from build123d import *

# Parameters (mm, degrees)
F0_R     = 10
F1_DEPTH = 1.5
F2_R     = 9
F3_DEPTH = 24
F4_R     = 7
F5_DEPTH = 25.501


with BuildPart() as f1:
    # F0 (on Top) → F1 (new body)
    with BuildSketch(Plane.XY):
        Circle(F0_R)
    extrude(amount=-F1_DEPTH)

    # F2 (on face) → F3 (join)
    with BuildSketch(Plane(origin=(0, 0, -1.5), x_dir=(1, 0, 0), z_dir=(0, 0, -1))):
        Circle(F2_R)
    extrude(amount=F3_DEPTH)

    # F4 (on face) → F5 (cut, through all)
    with BuildSketch(Plane.XY):
        Circle(F4_R)
    extrude(amount=-F5_DEPTH, mode=Mode.SUBTRACT)


solid = f1.part
Geometry: final body of the model. Coordinates: model frame, mm. Coordinates: 2 decimals unless noted, no trailing zeros. Order: outer loops, then holes, each group sorted by start corner. A loop starts at its lowest first (then second) coordinate and runs counter-clockwise, first axis right, second up. Notation, with made-up numbers: M 84.25,60.5 L 99.25,60.5 A18 ccw 99.25,70.5 Z; hole C 47.25,53.5 d2. An arc over 180 degrees is marked long. One line per question, with ' | ' between items. Start each with the question number.
Item 1: Cut plane C-C, the plane z = -8.5. Return the cut outline in (x, y), then the cut area to 3 significant figures.
Item 2: Cut plane B-B, the plane x = -4.25. Return the cut outline in (y, z).
Item 3: Ray query, probe 1 along Y at (x, z) = (0, -9); probe 2 along X at (y, z) = (5.5, -9.5); probe 3 along Z at (x, y) = (-9, 1). Return the intervals inside material, ascending. Write a range as [from, to].
Item 4: Pin query (flat end, axial travel): pin 1 Ø6 at (y, z) = (-3, -5.5) entering from +X; pin 2 Ø2 at (x, z) = (1.5, -8.5) entering from +Y; pin 3 Ø3 at (y, z) = (4.5, -11) entering from +X. Return the tip coordinate at first contact, or that it passes through.
Item 5: Draft query along Y for faces 1 (the flat face through (-9, 2, -1.5)), 2 (the cylindrical face through (-1.172, -8.923, -13.332)), 3 (the cylindrical face through (6.466, -2.681, -12.572)). Return one class per face: released by +Y, released by -Y, zero draft, split by the parting line, or undercut.
Item 6: Cut plane A-A, the plane y = 0. Return the cut outline in (x, z).
Item 7: Cut plane D-D, the plane x = 7.75. Return the cut outline in (y, z), then the cut area to 3 significant figures.
A:
1) outline: C 0,0 d18; hole C 0,0 d14 | area: 101 mm2
2) outline: M -9.05,-1.5 L -7.93,-1.5 L -7.93,-25.5 L -5.56,-25.5 L -5.56,0 L -9.05,0 Z; M 5.56,-25.5 L 7.93,-25.5 L 7.93,-1.5 L 9.05,-1.5 L 9.05,0 L 5.56,0 Z
3) probe 1: y = [-9, -7], [7, 9] | probe 2: x = [-7.12, -4.33], [4.33, 7.12] | probe 3: z = [-1.5, 0]
4) pin 1: stops at x = 9 | pin 2: stops at y = 8.99 | pin 3: stops at x = 8.49
5) face 1: zero draft | face 2: split by the parting line | face 3: undercut
6) outline: M -10,-1.5 L -9,-1.5 L -9,-25.5 L -7,-25.5 L -7,0 L -10,0 Z; M 7,-25.5 L 9,-25.5 L 9,-1.5 L 10,-1.5 L 10,0 L 7,0 Z
7) outline: M -6.32,-1.5 L -4.58,-1.5 L -4.58,-25.5 L 4.58,-25.5 L 4.58,-1.5 L 6.32,-1.5 L 6.32,0 L -6.32,0 Z | area: 239 mm2
